Read the model definition and answer for the solid it produces. Units are mm, in the model's axes. A direction names the side the tool comes from. Round coordinates to 2 decimals unless told otherwise and drop trailing zeros. Order: outer loops, then holes, each group sorted by start corner. A loop starts at its lowest first (then second) coordinate and runs counter-clockwise, first axis right, second up. Notation, with made-up numbers: (11, 87) -> (21, 87) arc R17 cw to (21, 119) -> close; hole circle Ø10 at (61, -23.75). An arc over 180 degrees is marked (long way). Answer as a JSON object with one key per item and string values. Group by question number.
Item 1: Given P1, Ø5, axis at x = -30, z = 25.5, coming from the -Y side; P2, Ø14, axis at x = 44.5, y = -33, coming from the -Z side; P3, Ø2, axis at x = -42.5, z = 25.5, coming from the +Y side, each flat-ended and moving along its own axis, determine where each tip first touches the part or whether it passes through.
Item 2: Section B-B, the plane z = 58.5 is taken. Write down the section's boundary in (x, y), plus the area to 3 significant figures.
Item 3: Section A-A, the plane z = 7 is taken. Write down the section's boundary in (x, y), plus the area to 3 significant figures.
Item 4: Section C-C, the plane y = -20 is taken. Write down the section's boundary in (x, z), plus the area to 3 significant figures.
Item 5: Consider probe 1 along Y at (x, z) = (0, 2.25); probe 2 along Z at (x, y) = (-29, -17); probe 3 along X at (y, z) = (56, 1). Determine where each line is inside the solid, lowest interval first. Write a range as from..to.
Item 6: For faces 1 (the flat face through (-44, -56, 3)), 2 (the flat face through (12.219, 0, 37)), 3 (the flat face through (50, -46, 33)), determine the directions among +Z, -Z, +X, -X, +Y, -Y from which every point of the face is accessible in a straight line to the end or side of a thin tool.
Item 7: The mould has two halves that part along Y. Classify faces 4 (the flat face through (37.254, 2.353, 38.059)), 5 (the flat face through (-25, -48, 22)), 6 (the flat face through (15, 0, 47)): pulls with the +Y half, pulls with the -Y half, needs draft (parallel to the pull), parting line crosses it, or undercut.
Item 8: Section D-D, the plane z = 32 is taken. Write down the section's boundary in (x, y), plus the area to 3 significant figures.
from build123d import *

# Parameters (mm, degrees)
SKETCH_R        = 1.5
SKETCH_R_2      = 10
PAD_DEPTH       = 3
SKETCH001_R     = 10
PAD001_DEPTH    = 60
SKETCH004_W     = 70
SKETCH004_H     = 25
POCKET_DEPTH    = 30
SKETCH005_W     = 70
SKETCH005_H     = 25
POCKET001_DEPTH = 30
SKETCH006_W     = 50
SKETCH006_H     = 25
POCKET002_DEPTH = 80
POCKET003_DEPTH = 13
SKETCH008_R     = 10
SKETCH008_R_2   = 3.5
PAD002_DEPTH    = 3
CHAMFER001_SIZE = 1
SKETCH009_R     = 1.5
POCKET004_DEPTH = 12
POCKET005_DEPTH = 10
POCKET006_DEPTH = 3.5
SKETCH012_W     = 30
SKETCH012_H     = 25
POCKET007_DEPTH = 1


with BuildPart() as part:
    # Sketch → Pad (new body)
    with BuildSketch(Plane.XY):
        with BuildLine():
            ThreePointArc((-9.0000068257, 66), (-14.8579724019, 64.1045764441), (-18.4952748867, 59.1368383489))
            Line((-55.4952734203, -52.8631572125), (-18.4952748867, 59.1368383489))
            ThreePointArc((-55.4952734203, -52.8631572125), (-47.58859463, -65.8730120582), (-36, -56))
            Line((-36, -56), (36, -56))
            ThreePointArc((36, -56), (47.5886025397, -65.8730107855), (55.4952683942, -52.8631419983))
            Line((18.4952730609, 59.1368438754), (55.4952683942, -52.8631419983))
            ThreePointArc((18.4952730609, 59.1368438754), (14.8579671858, 64.1045802143), (8.9999997739, 66))
            Line((-9.0000068257, 66), (8.9999997739, 66))
        make_face()
        with Locations((-9, 56)):
            Circle(SKETCH_R, mode=Mode.SUBTRACT)
        with Locations((9, 56)):
            Circle(SKETCH_R, mode=Mode.SUBTRACT)
        with Locations((-46, -56)):
            Circle(SKETCH_R, mode=Mode.SUBTRACT)
        with Locations((46, -56)):
            Circle(SKETCH_R, mode=Mode.SUBTRACT)
        Circle(SKETCH_R_2, mode=Mode.SUBTRACT)
        with Locations((0, 56)):
            Circle(SKETCH_R, mode=Mode.SUBTRACT)
    extrude(amount=PAD_DEPTH)

    # Sketch001 (on Face16 of Pad) → Pad001 (join)
    with BuildSketch(Plane.XY.offset(3)):
        with BuildLine():
            ThreePointArc((-36, -56), (-38.9289322782, -48.9289320981), (-46.0000002547, -46))
            Line((-53.2279804126, -46), (-46.0000002547, -46))
            Line((-22.8351232698, 46), (-53.2279804126, -46))
            Line((-22.8351232698, 46), (22.8351232698, 46))
            Line((53.2279804126, -46), (22.8351232698, 46))
            Line((45.999999471, -46), (53.2279804126, -46))
            ThreePointArc((45.999999471, -46), (38.9289320011, -48.9289323752), (36, -56))
            Line((-36, -56), (36, -56))
        make_face()
        Circle(SKETCH001_R, mode=Mode.SUBTRACT)
    extrude(amount=PAD001_DEPTH)

    # Sketch004 (on Face25 of Pad001) → Pocket (cut)
    with BuildSketch(Plane(origin=(34.2893542942, 11.3277331151, 0), x_dir=(-0.3136832519, 0.9495276813, 0), z_dir=(0.9495276813, 0.3136832519, 0))):
        with Locations((-10, 22.5)):
            Rectangle(SKETCH004_W, SKETCH004_H)
    extrude(amount=-POCKET_DEPTH, mode=Mode.SUBTRACT)

    # Sketch005 (on Face9 of Pocket) → Pocket001 (cut)
    with BuildSketch(Plane(origin=(-34.2893542942, 11.3277331151, 0), x_dir=(-0.3136832519, -0.9495276813, 0), z_dir=(-0.9495276813, 0.3136832519, 0))):
        with Locations((10, 22.5)):
            Rectangle(SKETCH005_W, SKETCH005_H)
    extrude(amount=-POCKET001_DEPTH, mode=Mode.SUBTRACT)

    # Sketch006 (on Face27 of Pocket001) → Pocket002 (cut)
    with BuildSketch(Plane.XZ.offset(56)):
        with Locations((0, 22.5)):
            Rectangle(SKETCH006_W, SKETCH006_H)
    extrude(amount=-POCKET002_DEPTH, mode=Mode.SUBTRACT)

    # Sketch007 (on Face22 of Pocket002) → Pocket003 (cut)
    with BuildSketch(Plane.XY.offset(63)):
        with BuildLine():
            ThreePointArc((6.5, -51.5921505658), (0, 52), (-6.5, -51.5921505658))
            Line((-6.5, -51.5921505658), (-6.5, -56.5921505658))
            Line((6.5, -56.5921505658), (-6.5, -56.5921505658))
            Line((6.5, -51.5921505658), (6.5, -56.5921505658))
        make_face()
    extrude(amount=-POCKET003_DEPTH, mode=Mode.SUBTRACT)

    # Sketch008 → Pad002 (join)
    with BuildSketch(Plane.XY.offset(50)):
        Circle(SKETCH008_R)
        Circle(SKETCH008_R_2, mode=Mode.SUBTRACT)
    extrude(amount=-PAD002_DEPTH)

    # Chamfer001
    chamfer001_edges = [part.edges().sort_by_distance(p)[0] for p in [
        (7.5, 56, 3),
        (-10.5, 56, 3),
        (-1.5, 56, 0),
    ]]
    chamfer(chamfer001_edges, length=CHAMFER001_SIZE)

    # Sketch009 → Pocket004 (cut)
    with BuildSketch(Plane(origin=(0, 0, 35), x_dir=(1, 0, 0), z_dir=(0, 0, -1))):
        with Locations((-15.25, 0)):
            Circle(SKETCH009_R)
        with Locations((15.25, 0)):
            Circle(SKETCH009_R)
    extrude(amount=-POCKET004_DEPTH, mode=Mode.SUBTRACT)

    # Sketch010 → Pocket005 (cut)
    with BuildSketch(Plane(origin=(0, 0, 0), x_dir=(1, 0, 0), z_dir=(0, 0, -1))):
        with BuildLine():
            ThreePointArc((-12.4999765902, 10), (-22.5, 2e-10), (-12.4999765905, -10))
            Line((12.4999765907, -10), (-12.4999765905, -10))
            ThreePointArc((12.4999765907, -10), (22.5, 4e-10), (12.49997659, 10))
            Line((-12.4999765902, 10), (12.49997659, 10))
        make_face()
    extrude(amount=-POCKET005_DEPTH, mode=Mode.SUBTRACT)

    # Sketch011 (on Face62 of Pocket005) → Pocket006 (cut)
    with BuildSketch(Plane(origin=(0, 0, 35), x_dir=(1, 0, 0), z_dir=(0, 0, -1))):
        Polygon((-15.25, 3.5), (-18.2810889132, 1.75), (-18.2810889132, -1.75), (-15.25, -3.5), (-12.2189110868, -1.75), (-12.2189110868, 1.75), align=None)
        Polygon((15.25, 3.5), (12.2189110868, 1.75), (12.2189110868, -1.75), (15.25, -3.5), (18.2810889132, -1.75), (18.2810889132, 1.75), align=None)
    extrude(amount=-POCKET006_DEPTH, mode=Mode.SUBTRACT)

    # Sketch012 (on Face1 of Pocket006) → Pocket007 (cut)
    with BuildSketch(Plane(origin=(0, 0, 0), x_dir=(1, 0, 0), z_dir=(0, 0, -1))):
        with Locations((-50, 30.5)):
            Rectangle(SKETCH012_W, SKETCH012_H)
        with Locations((50, 30.5)):
            Rectangle(SKETCH012_W, SKETCH012_H)
    extrude(amount=-POCKET007_DEPTH, mode=Mode.SUBTRACT)


solid = part.part
Values found:
{
 "1": {"P1": "y = -56", "P2": "z = 1", "P3": "y = -33.02"},
 "2": {"outline": "(-53.23, -46) -> (-46, -46) arc R10 cw to (-36, -56) -> (-6.5, -56) -> (-6.5, -51.59) arc R52 cw to (-46.03, -24.2) -> close; (6.5, -56) -> (36, -56) arc R10 cw to (46, -46) -> (53.23, -46) -> (46.03, -24.2) arc R52 cw to (6.5, -51.59) -> close", "area": "1,050 mm2"},
 "3": {"outline": "(-53.23, -46) -> (-46, -46) arc R10 cw to (-36, -56) -> (36, -56) arc R10 cw to (46, -46) -> (53.23, -46) -> (22.84, 46) -> (-22.84, 46) -> close; hole (-12.5, -10) -> (12.5, -10) arc R10 ccw to (12.5, 10) -> (-12.5, 10) arc R10 ccw to start", "area": "6,950 mm2"},
 "4": {"outline": "(-44.64, 1) -> (-35, 1) -> (-35, 0) -> (35, 0) -> (35, 1) -> (44.64, 1) -> (44.64, 10) -> (-44.64, 10) -> close; (-44.64, 35) -> (44.64, 35) -> (44.64, 50) -> (-44.64, 50) -> close", "area": "2,210 mm2"},
 "5": {"probe 1": "-56..-10, 10..54.5, 57.5..66", "probe 2": "0..10, 35..50", "probe 3": "-19.53..-10.5, -7.5..-1.5, 1.5..7.5, 10.5..19.53"},
 "6": {"face 1": "+Z, -X, -Y", "face 2": "-Z", "face 3": "+Z, +X, -Y"},
 "7": {"face 4": "pulls with the +Y half", "face 5": "needs draft", "face 6": "undercut"},
 "8": {"outline": "(-53.23, -46) -> (-46, -46) arc R10 cw to (-36, -56) -> (-25, -56) -> (-25, -39.13) -> (-48.41, -31.4) -> close; (-26.45, 35.07) -> (0, 26.33) -> (26.45, 35.07) -> (22.84, 46) -> (-22.84, 46) -> close; (25, -56) -> (36, -56) arc R10 cw to (46, -46) -> (53.23, -46) -> (48.41, -31.4) -> (25, -39.13) -> close", "area": "1,610 mm2"}
}
